from build123d import *

# Parameters (mm, degrees)
SKETCH_1_W          = 70
SKETCH_1_H          = 70
EXTRUDE_1_DEPTH     = 2.8
SKETCH_2_W          = 30
SKETCH_2_H          = 30
CUT_EXTRUDE_1_DEPTH = 2
SKETCH_3_R          = 2.6
CUT_EXTRUDE_2_DEPTH = 3
EXTRUDE_2_DEPTH     = 2.3
SKETCH_6_R          = 1.6
EXTRUDE_3_DEPTH     = 0.3


with BuildPart() as part:
    # 草图1 → 凸台-拉伸1 (new body)
    with BuildSketch(Plane.XY):
        with BuildLine():
            Line((-2, 17), (0, 17))
            Line((0, 17), (0, 53))
            Line((0, 53), (-2, 53))
            ThreePointArc((-2, 53), (-4.121320344, 52.121320344), (-5, 50))
            Line((-5, 50), (-5, 20))
            ThreePointArc((-5, 20), (-4.121320344, 17.878679656), (-2, 17))
        make_face()
        with Locations((35, 35)):
            Rectangle(SKETCH_1_W, SKETCH_1_H)
        with BuildLine():
            Line((70, 53), (70, 17))
            Line((70, 17), (72, 17))
            ThreePointArc((72, 17), (74.121320344, 17.878679656), (75, 20))
            Line((75, 20), (75, 50))
            ThreePointArc((75, 50), (74.121320344, 52.121320344), (72, 53))
            Line((72, 53), (70, 53))
        make_face()
    extrude(amount=EXTRUDE_1_DEPTH)

    # 草图2 → 切除-拉伸1 (cut)
    with BuildSketch(Plane.XY.offset(2.8)):
        with Locations((35, 35)):
            Rectangle(SKETCH_2_W, SKETCH_2_H)
    extrude(amount=-CUT_EXTRUDE_1_DEPTH, mode=Mode.SUBTRACT)

    # 草图3 → 切除-拉伸2 (cut)
    with BuildSketch(Plane.XY.offset(2.8)):
        with Locations((8, 62)):
            Circle(SKETCH_3_R)
        with Locations((62, 62)):
            Circle(SKETCH_3_R)
        with Locations((8, 8)):
            Circle(SKETCH_3_R)
        with Locations((62, 8)):
            Circle(SKETCH_3_R)
    extrude(amount=-CUT_EXTRUDE_2_DEPTH, mode=Mode.SUBTRACT)

    # 草图4 → 凸台-拉伸2 (add)
    with BuildSketch(Plane.XY):
        with BuildLine():
            Line((20, 44), (20, 50))
            Line((20, 50), (26, 50))
            ThreePointArc((26, 50), (24.242640687, 45.757359313), (20, 44))
        make_face()
        with BuildLine():
            Line((50, 44), (50, 50))
            Line((50, 50), (44, 50))
            ThreePointArc((44, 50), (45.757359313, 45.757359313), (50, 44))
        make_face()
        with BuildLine():
            Line((50, 20), (44, 20))
            ThreePointArc((44, 20), (45.757359313, 24.242640687), (50, 26))
            Line((50, 26), (50, 20))
        make_face()
        with BuildLine():
            Line((20, 26), (20, 20))
            Line((20, 20), (26, 20))
            ThreePointArc((26, 20), (24.242640687, 24.242640687), (20, 26))
        make_face()
    extrude(amount=EXTRUDE_2_DEPTH)

    # 草图6 → 凸台-拉伸3 (add)
    with BuildSketch(Plane.XY.offset(2.3)):
        with Locations((22.5, 47.5)):
            Circle(SKETCH_6_R)
        with Locations((47.5, 47.5)):
            Circle(SKETCH_6_R)
        with Locations((47.5, 22.5)):
            Circle(SKETCH_6_R)
        with Locations((22.5, 22.5)):
            Circle(SKETCH_6_R)
        Polygon((20.1, 45.5), (20.7, 45.5), (20.7, 46.1), (21.3, 46.1), (21.3, 45.5), (21.9, 45.5), (21.9, 44.9), (21.3, 44.9), (21.3, 44.3), (20.7, 44.3), (20.7, 44.9), (20.1, 44.9), align=None)
    extrude(amount=EXTRUDE_3_DEPTH)


solid = part.part
Model file for the job. Use its own axes, mm. A direction names the side the tool comes from. Give positions to 0.01 mm unless a question says otherwise; leave off trailing zeros. Order: outer loops, then holes, each group sorted by start corner. A loop starts at its lowest first (then second) coordinate and runs counter-clockwise, first axis right, second up. Notation, with made-up numbers: (24.5, 29.5) - (80.5, 29.5) arc R13 cw to (80.5, 44.5) - close; hole circle Ø10 at (-7.5, 60.5). An arc over 180 degrees is marked (long way). Write item = value, one per line. Start each with the question number.
1. Two-plate mould, pull along X, no slides. Class faces 1 (the cylindrical face through (74.1, 17.86, 1.38)), 2 (the cylindrical face through (-4.1, 52.14, 1.38)), 3 (the flat face through (24, 24, 2.3)), 4 (the flat face through (52, 35, 2.8)): pulls with the +X half, pulls with the -X half, needs draft (parallel to the pull), parting line crosses it, or undercut.
2. Which spindle directions (+Z, -Z, +X, -X, +Y, -Y) get a long thin tool onto all of the face, cutting with end or side? Do faces 5 (the cylindrical face through (59.4, 62.1, 1.4)), 6 (the flat face through (47, 23, 2.6)), 7 (the flat face through (-1, 53, 1)). Say none if no direction does.
3. Drop flat-ended pins along their axis: P1, Ø1.8, axis at x = 22, y = 48.5, coming from the +Z side; P2, Ø0.8, axis at y = 58.5, z = 2, coming from the -X side; P3, Ø1.5, axis at x = 47, y = 42, coming from the +Z side. Give the stop position or say it passes through.
4. Probe line 1 along Y through (x, z) = (62, 1.7); line 2 along Y through (x, z) = (9, 1.05); line 3 along X through (y, z) = (6.5, 0.9). List the from-to ranges inside material, lowest first.
5. Cut at A-A, the plane z = 1.25. List the corners of the cut face in (x, y), and give its area (3 significant figures).
6. Cut at D-D, the plane y = 38. List the corners of the cut face in (x, z), and give its area (3 significant figures).
7. Cut at B-B, the plane y = 8. List the corners of the cut face in (x, z), and give its area (3 significant figures).
Taken from the geometry:
q1.face_1 = pulls with the +X half
q1.face_2 = pulls with the -X half
q1.face_3 = undercut
q1.face_4 = needs draft
q2.face_5 = +Z, -Z
q2.face_6 = +Z
q2.face_7 = +Z, -Z, -X, +Y
q3.P1 = 2.6
q3.P2 = 0
q3.P3 = 0.8
q4.line_1 = 0 to 5.4, 10.6 to 59.4, 64.6 to 70
q4.line_2 = 0 to 5.6, 10.4 to 59.6, 64.4 to 70
q4.line_3 = 0 to 5.88, 10.12 to 59.88, 64.12 to 70
q5.outline = (-5, 20) arc R3 ccw to (-2, 17) - (0, 17) - (0, 0) - (70, 0) - (70, 17) - (72, 17) arc R3 ccw to (75, 20) - (75, 50) arc R3 ccw to (72, 53) - (70, 53) - (70, 70) - (0, 70) - (0, 53) - (-2, 53) arc R3 ccw to (-5, 50) - close; hole circle Ø5.2 at (8, 8); hole circle Ø5.2 at (8, 62); hole (20, 26) arc R6 cw to (26, 20) - (44, 20) arc R6 cw to (50, 26) - (50, 44) arc R6 cw to (44, 50) - (26, 50) arc R6 cw to (20, 44) - close; hole circle Ø5.2 at (62, 8); hole circle Ø5.2 at (62, 62)
q5.area = 4,380 mm²
q6.outline = (-5, 0) - (75, 0) - (75, 2.8) - (50, 2.8) - (50, 0.8) - (20, 0.8) - (20, 2.8) - (-5, 2.8) - close
q6.area = 164 mm²
q7.outline = (0, 0) - (5.4, 0) - (5.4, 2.8) - (0, 2.8) - close; (10.6, 0) - (59.4, 0) - (59.4, 2.8) - (10.6, 2.8) - close; (64.6, 0) - (70, 0) - (70, 2.8) - (64.6, 2.8) - close
q7.area = 167 mm²
